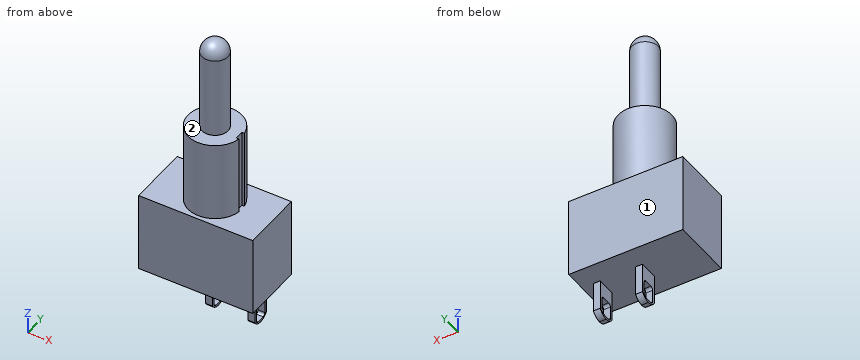
```python
from build123d import *

# Parameters (mm, degrees)
F0_W      = 12.7
F0_H      = 6.86
F1_DEPTH  = 8.89
F2_R      = 3
F3_DEPTH  = 8.89
F4_R      = 1.46
F5_DEPTH  = 10.5
F6_R      = 1.46
F7_W      = 0.434782
F7_H      = 1
F8_DEPTH  = 25
F9_W      = 0.76
F9_H      = 2.1
F10_DEPTH = 3.94
F12_DEPTH = 11.431


with BuildPart() as f1:
    # F0 (on Top) → F1 (new body)
    with BuildSketch(Plane.XY):
        Rectangle(F0_W, F0_H)
    extrude(amount=-F1_DEPTH)

    # F2 (on Top) → F3 (join)
    with BuildSketch(Plane.XY):
        Circle(F2_R)
    extrude(amount=F3_DEPTH)

    # F4 (on face) → F5 (join)
    with BuildSketch(Plane.XY.offset(8.89)):
        Circle(F4_R)
    extrude(amount=F5_DEPTH)

    # F6
    f6_edges = [f1.edges().sort_by_distance(p)[0] for p in [
        (-1.46, 0, 19.39),
    ]]
    fillet(f6_edges, radius=F6_R)

    # F7 (on Top) → F8 (cut)
    with BuildSketch(Plane.XY):
        with Locations((2.9, 0)):
            Rectangle(F7_W, F7_H)
    extrude(amount=F8_DEPTH, mode=Mode.SUBTRACT)

    # F9 (on face) → F10 (join)
    with BuildSketch(Plane(origin=(0, 0, -8.89), x_dir=(1, 0, 0), z_dir=(0, 0, -1))):
        Rectangle(F9_W, F9_H)
        with Locations((4.7, 0)):
            Rectangle(F9_W, F9_H)
    extrude(amount=F10_DEPTH)

    # F11 (on face) → F12 (cut, through all)
    with BuildSketch(Plane.YZ.offset(5.08)):
        with BuildLine():
            Line((0.45, -10.53), (-0.45, -10.53))
            ThreePointArc((-0.45, -10.53), (-0.662132, -10.617868), (-0.75, -10.83))
            Line((-0.75, -10.83), (-0.75, -12.23))
            ThreePointArc((-0.75, -12.23), (-0.662132, -12.442132), (-0.45, -12.53))
            Line((-0.45, -12.53), (0.45, -12.53))
            ThreePointArc((0.45, -12.53), (0.662132, -12.442132), (0.75, -12.23))
            Line((0.75, -12.23), (0.75, -10.83))
            ThreePointArc((0.75, -10.83), (0.662132, -10.617868), (0.45, -10.53))
        make_face()
        with BuildLine():
            ThreePointArc((1.05, -12.23), (0.604669, -12.669421), (0, -12.83))
            Line((0, -12.83), (1.05, -12.83))
            Line((1.05, -12.83), (1.05, -12.23))
        make_face()
        with BuildLine():
            ThreePointArc((0, -12.83), (-0.604669, -12.669421), (-1.05, -12.23))
            Line((-1.05, -12.23), (-1.05, -12.83))
            Line((-1.05, -12.83), (0, -12.83))
        make_face()
    extrude(amount=-F12_DEPTH, mode=Mode.SUBTRACT)


solid = f1.part
```
The listing builds one solid part. Answer for the finished solid, in the listing's coordinates (mm). Face numbers are marked on the shaded views. A direction names the side the tool comes from. Give positions to 0.01 mm unless a question says otherwise; leave off trailing zeros. Write each loop counter-clockwise with the first axis right and the second up, starting at its lowest first coordinate (ties: lowest second). Pieces come first, ordered by that corner, then holes. Notation, with made-up numbers: (79.25, 43.5) - (99.25, 43.5) arc R31 ccw to (99.25, 80.5) - close; hole circle Ø3 at (46.5, -29). An arc over 180 degrees is marked (long way). Use one line per item in the form item = value. Start each with the question number.
1) Find section C-C on x = -2.5. Determine the outline of the cut face in (y, z).
2) Consider line 1 along Z through (x, y) = (5.25, -0.5); line 2 along Z through (x, y) = (-0.25, -2.5); line 3 along Y through (x, z) = (2.75, 2). Determine where each line is inside the solid, lowest interval first. Write a range as from..to.
3) Find section D-D on z = 12. Determine the outline of the cut face in (x, y), plus the area to 3 significant figures.
4) Find section A-A on x = 0. Determine the outline of the cut face in (y, z), plus the area to 3 significant figures.
5) A tool of negligible diameter and unlimited length cuts with its end or side. For the marked faces 1 and 2, from which of +Z, -Z, +X, -X, +Y, -Y can it reach the whole face along a straight path? Write none if from no direction.
6) Flat-ended cylindrical pins translate along their axes: pin 1 Ø0.5 at (y, z) = (0, 3.5) entering from +X; pin 2 Ø0.8 at (x, z) = (0, -10.5) entering from -Y; pin 3 Ø1.7 at (y, z) = (0, -11.5) entering from +X. Find the tip coordinate at first contact, or state that the pin passes through.
7) Find section B-B on z = 1.5. Determine the outline of the cut face in (x, y).
Geometry results:
q1.outline = (-3.43, -8.89) - (3.43, -8.89) - (3.43, 0) - (1.66, 0) - (1.66, 8.89) - (-1.66, 8.89) - (-1.66, 0) - (-3.43, 0) - close
q2.line_1 = -8.89..0
q2.line_2 = -8.89..8.89
q2.line_3 = -1.2..-0.5, 0.5..1.2
q3.outline = circle Ø2.92 at (0, 0)
q3.area = 6.70 mm2
q4.outline = (-3.43, -8.89) - (-1.05, -8.89) - (-1.05, -12.23) arc R1.22 ccw to (0, -12.83) arc R1.22 ccw to (1.05, -12.23) - (1.05, -8.89) - (3.43, -8.89) - (3.43, 0) - (3, 0) - (3, 8.89) - (1.46, 8.89) - (1.46, 17.93) arc R1.46 ccw to (-1.46, 17.93) - (-1.46, 8.89) - (-3, 8.89) - (-3, 0) - (-3.43, 0) - close; hole (-0.75, -12.23) arc R0.3 ccw to (-0.45, -12.53) - (0.45, -12.53) arc R0.3 ccw to (0.75, -12.23) - (0.75, -10.83) arc R0.3 ccw to (0.45, -10.53) - (-0.45, -10.53) arc R0.3 ccw to (-0.75, -10.83) - close
q4.area = 149 mm2
q5.face_1 = +Z, -Z, +X, -X, +Y
q5.face_2 = +Z
q6.pin_1 = 2.68
q6.pin_2 = -1.05
q6.pin_3 = 5.08
q7.outline = (2.68, -0.5) - (2.68, 0.5) - (2.96, 0.5) arc R3 ccw (long way) to (2.96, -0.5) - close
